Autodesk Inventor part; units mm, degrees
ref_plane "YZ Plane" through (0, 0, 0) normal (1, 0, 0) x (0, 1, 0)
ref_plane "XZ Plane" through (0, 0, 0) normal (0, 1, 0) x (-1, 0, 0)
ref_plane "XY Plane" through (0, 0, 0) normal (0, 0, 1) x (1, 0, 0)
sketch "Boceto1" plane through (0, 0, 0) normal (0, 0, 1) x (1, 0, 0)
  arc A0 (-116.1173, -7.6512) -> (-117.6673, -9.2012) centre (-116.1173, -9.2012) ccw
  arc A1 (-117.6673, -9.2012) -> (-116.1173, -10.7512) centre (-116.1173, -9.2012) ccw
  arc A2 (-116.1173, -10.7512) -> (-114.5673, -9.2012) centre (-116.1173, -9.2012) ccw
  arc A3 (-114.5673, -9.2012) -> (-116.1173, -7.6512) centre (-116.1173, -9.2012) ccw
  arc A4 (-116.1173, -36.6512) -> (-117.6673, -38.2012) centre (-116.1173, -38.2012) ccw
  arc A5 (-117.6673, -38.2012) -> (-116.1173, -39.7512) centre (-116.1173, -38.2012) ccw
  arc A6 (-116.1173, -39.7512) -> (-114.5673, -38.2012) centre (-116.1173, -38.2012) ccw
  arc A7 (-114.5673, -38.2012) -> (-116.1173, -36.6512) centre (-116.1173, -38.2012) ccw
  arc A8 (-107.1173, -22.7512) -> (-112.0673, -27.7012) centre (-107.1173, -27.7012) ccw
  arc A9 (-112.0673, -27.7012) -> (-107.1173, -32.6512) centre (-107.1173, -27.7012) ccw
  arc A10 (-107.1173, -32.6512) -> (-102.1673, -27.7012) centre (-107.1173, -27.7012) ccw
  arc A11 (-102.1673, -27.7012) -> (-107.1173, -22.7512) centre (-107.1173, -27.7012) ccw
  line L0 (-122.3173, 0.4988) -> (-122.3173, -42.9012)
  line L1 (-122.3173, -42.9012) -> (-80.1673, -42.9012)
  line L2 (-80.1673, -42.9012) -> (-80.1673, -32.9643)
  line L3 (-80.1673, -32.9643) -> (-91.9173, -32.9643)
  line L4 (-91.9173, -32.9643) -> (-91.9173, -15.4172)
  line L5 (-91.9173, -15.4172) -> (-80.1673, -15.4172)
  line L6 (-80.1673, -15.4172) -> (-80.1673, 0.4988)
  line L7 (-80.1673, 0.4988) -> (-83.3173, 0.4988)
  line L8 (-83.3173, 0.4988) -> (-83.3173, -2.0012)
  line L9 (-83.3173, -2.0012) -> (-111.9173, -2.0012)
  line L10 (-111.9173, -2.0012) -> (-111.9173, 0.4988)
  line L11 (-111.9173, 0.4988) -> (-122.3173, 0.4988)
  point P0 (0, 0)
extrude "Extrusión1" add sketch "Boceto1" along normal blind 5
properties part number "carro x lado motor pieza 2parte 2"
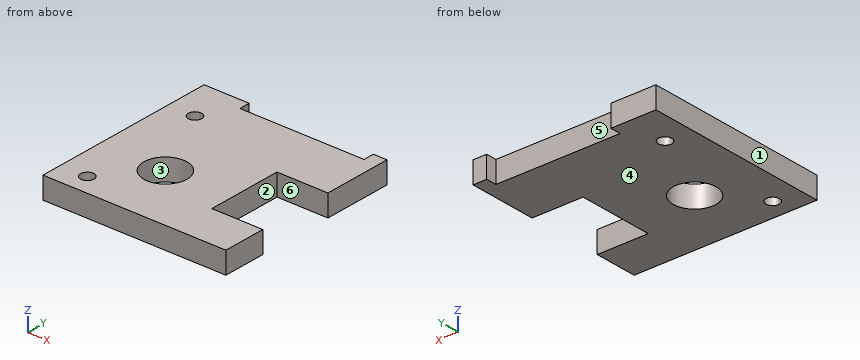
Model file for the job. Use its own axes, mm. Face numbers are marked on the shaded views. A direction names the side the tool comes from. Give positions to 0.01 mm unless a question says otherwise; leave off trailing zeros. Loops run counter-clockwise (first coordinate to the right, second up) from the corner with the lowest first, then second, coordinate; pieces in that order, holes last. Notation, with made-up numbers: M 1,-37.5 L 58,-37.5 A28 cw 58,-0.5 Z; hole C 69,83 d8. An arc over 180 degrees is marked long. Use one line per item in the form item = value.
Item 1: Slice it at C-C on z = 1.95. List the corners of the cut face in (x, y).
Filled in:
outline = M -122.32,-42.9 L -80.17,-42.9 L -80.17,-32.96 L -91.92,-32.96 L -91.92,-15.42 L -80.17,-15.42 L -80.17,0.5 L -83.32,0.5 L -83.32,-2 L -111.92,-2 L -111.92,0.5 L -122.32,0.5 Z; hole C -116.12,-38.2 d3.1; hole C -116.12,-9.2 d3.1; hole C -107.12,-27.7 d9.9
Item 2: Two-plate mould, pull along X, no slides. Class the marked faces 1, 2 and 3: released by +X, released by -X, zero draft, split by the parting line, or undercut.
Filled in:
face_1 = released by -X
face_2 = released by +X
face_3 = undercut
Item 3: Drill centre lines: L1, parallel to Y at x = -86, z = 1.7; L2, parallel to Y at x = -117, z = 0.6; L3, parallel to X at y = -21, z = 0.5. Where is each one in solid material? Low to high.
Filled in:
L1 = -42.9 to -32.96, -15.42 to -2
L2 = -42.9 to -39.48, -36.93 to -10.48, -7.93 to 0.5
L3 = -122.32 to -91.92
Item 4: Slice it at D-D on x = -93. List the corners of the cut face in (y, z), and give its area (4 significant figures).
Filled in:
outline = M -42.9,0 L -2,0 L -2,5 L -42.9,5 Z
area = 204.5 mm^2
Item 5: Flat gauge pins, fed straight in: pin 1 Ø1 at (y, z) = (-29, 3) entering from +X; pin 2 Ø2.5 at (x, z) = (-90.5, 3.5) entering from +Y. Where does each tip first touch, or does it go through?
Filled in:
pin_1 = -91.92
pin_2 = -2
Item 6: Slice it at B-B on y = -23.5. List the corners of the cut face in (x, z).
Filled in:
outline = M -122.32,0 L -109.74,0 L -109.74,5 L -122.32,5 Z; M -104.5,0 L -91.92,0 L -91.92,5 L -104.5,5 Z
Item 7: Which spindle directions (+Z, -Z, +X, -X, +Y, -Y) get a long thin tool onto all of the face, cutting with end or side? Do the marked faces 4, 5 and 6. Say none if no direction does.
Filled in:
face_4 = -Z, +X, -X, +Y, -Y
face_5 = +Z, -Z, +Y
face_6 = +Z, -Z, +X
Item 8: Slice it at A-A on x = -84. List the corners of the cut face in (y, z).
Filled in:
outline = M -42.9,0 L -32.96,0 L -32.96,5 L -42.9,5 Z; M -15.42,0 L -2,0 L -2,5 L -15.42,5 Z
